CAD build for the part. Positions are in the model's coordinates, mm. Face numbers are marked on the shaded views. A direction names the side the tool comes from. Round coordinates to 2 decimals unless told otherwise and drop trailing zeros. Order: outer loops, then holes, each group sorted by start corner. A loop starts at its lowest first (then second) coordinate and runs counter-clockwise, first axis right, second up. Notation, with made-up numbers: (88, 88) -> (96, 88) arc R20 ccw to (96, 111) -> close; hole circle Ø7 at (81.25, 40.25). An arc over 180 degrees is marked (long way). Return JSON: item names as keys, results as strings. Group by question number.
Q1. Cut at B-B (z = 175). Write the cut outline in (x, y).
Q2. Cut at D-D (y = 35.5). Write the cut outline in (x, z).
Q3. Which spindle directions (+Z, -Z, +X, -X, +Y, -Y) get a long thin tool onto all of the face, cutting with end or side? Do the marked faces 1 and 2. Say none if no direction does.
Q4. Probe line 1 along Z through (x, y) = (81.5, 26.5); line 2 along Z through (x, y) = (73, 26); line 3 along Z through (x, y) = (8.5, 20.5). List the from-to ranges inside material, lowest first.
Q5. Cut at C-C (x = 56). Write the cut outline in (y, z), then the cut area to 3 significant figures.
Q6. Cut at A-A (z = 201.5). Write the cut outline in (x, y).
Q7. Flat gauge pins, fed straight in: pin 1 (3 mm diameter, centred on y = 29, z = 156.5, fed in from +X); pin 2 (1.5 mm diameter, centred on x = 9, y = 27, fed in from +Z); pin 3 (2 mm diameter, centred on x = 36, z = 187.5, fed in from -Y). Where does each tip first touch, or does it go through?
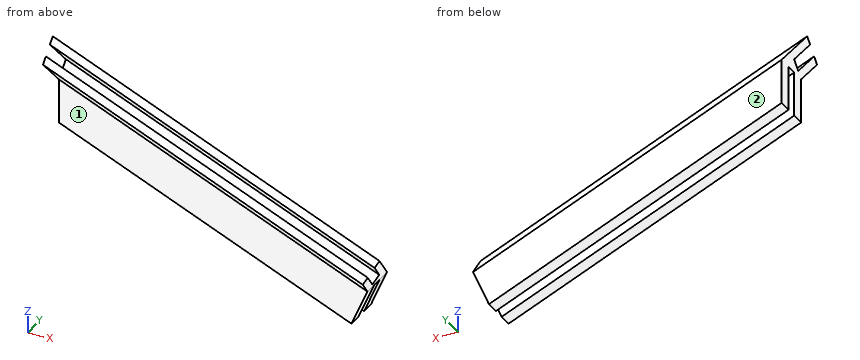
from build123d import *

# Parameters (mm, degrees)
SKETCH1_W           = 214.089522673
SKETCH1_H           = 271.033566845
BOSS_EXTRUDE1_DEPTH = 10
SKETCH3_W           = 107.044761337
SKETCH3_H           = 271.033566845
CUT_EXTRUDE1_DEPTH  = 252.253590179
CUT_EXTRUDE2_DEPTH  = 249.55642867
BOSS_EXTRUDE3_DEPTH = 40
CUT_EXTRUDE3_START  = -165.689856025
CUT_EXTRUDE3_DEPTH  = 205.862728092
CUT_EXTRUDE4_DEPTH  = 250.960593361
CUT_EXTRUDE5_DEPTH  = 250.960593361
CUT_EXTRUDE11_DEPTH = 252.67545035
SKETCH26_W          = 104.148686
SKETCH26_H          = 11.3
BOSS_EXTRUDE7_DEPTH = 45
CUT_EXTRUDE12_DEPTH = 250.816831154
CUT_EXTRUDE13_DEPTH = 252.67545035
CUT_EXTRUDE14_DEPTH = 237.436663672


with BuildPart() as part:
    # Sketch1 → Boss-Extrude1 (new body)
    with BuildSketch(Plane(origin=(0, 0, 0), x_dir=(1, 0, 0), z_dir=(0, 1, 0))):
        with Locations((-3.148375333, -90.062114546)):
            Rectangle(SKETCH1_W, SKETCH1_H)
    extrude(amount=BOSS_EXTRUDE1_DEPTH)

    # Sketch3 → Cut-Extrude1 (cut, through all)
    with BuildSketch(Plane(origin=(0, 10, 0), x_dir=(1, 0, 0), z_dir=(0, 1, 0))):
        with Locations((-56.670756002, -90.062114546)):
            Rectangle(SKETCH3_W, SKETCH3_H)
    extrude(amount=-CUT_EXTRUDE1_DEPTH, mode=Mode.SUBTRACT)

    # Sketch4 → Cut-Extrude2 (cut, through all)
    with BuildSketch(Plane(origin=(0, 10, 0), x_dir=(1, 0, 0), z_dir=(0, 1, 0))):
        Polygon((103.896386003, -181.239506042), (100.834918545, -173.848469781), (9.996584241, 45.454668877), (103.896386003, 45.454668877), align=None)
    extrude(amount=-CUT_EXTRUDE2_DEPTH, mode=Mode.SUBTRACT)

    # Sketch6 → Boss-Extrude3 (add, along a direction that is not the sketch's normal)
    with BuildSketch(Plane(origin=(0, 10, 0), x_dir=(1, 0, 0), z_dir=(0, 1, 0))):
        Polygon((99.572063218, -170.799667324), (103.896386003, -181.239506042), (-3.148375333, -225.578897968), (-3.148375333, -213.347866105), align=None)
    extrude(amount=BOSS_EXTRUDE3_DEPTH, dir=(-0.2705980500730979, 0.7071067811865489, -0.6532814824381872))

    # Cut-Extrude3: read off the stored shape, not the designer's step
    # Cut-Extrude3 outline → Cut-Extrude3 (cut)
    with BuildSketch(Plane(origin=(0, 0, 0), x_dir=(1, 0, 0), z_dir=(0, 0.6785983445458481, -0.7345095552677544)).offset(CUT_EXTRUDE3_START)):
        Polygon((-3.148375333, -165), (-3.148375333, -152.122604304), (-13.972297336, -155.165042499), (-15, -155.45391393), (-15, -165), align=None)
    extrude(amount=CUT_EXTRUDE3_DEPTH, mode=Mode.SUBTRACT)

    # Sketch8 → Cut-Extrude4 (cut, through all)
    with BuildSketch(Plane(origin=(0, 10, 0), x_dir=(1, 0, 0), z_dir=(0, 1, 0))):
        Polygon((-3.148375333, -225.578897968), (103.896386003, -181.239506042), (103.896386003, -225.578897968), align=None)
    extrude(amount=-CUT_EXTRUDE4_DEPTH, mode=Mode.SUBTRACT)

    # Sketch9 → Cut-Extrude5 (cut, through all)
    with BuildSketch(Plane(origin=(0, 10, 0), x_dir=(1, 0, 0), z_dir=(0, 1, 0))):
        Polygon((-3.148375333, -213.347866105), (99.572063218, -170.799667324), (9.996584241, 45.454668877), (-3.148375333, 45.454668877), align=None)
    extrude(amount=-CUT_EXTRUDE5_DEPTH, mode=Mode.SUBTRACT)

    # Sketch25 → Cut-Extrude11 (cut, through all)
    with BuildSketch(Plane(origin=(24.603270673, 0, -10.191008392), x_dir=(-0.38268343236508967, 0, -0.9238795325112868), z_dir=(0.9238795325112867, 0, -0.3826834323650896))):
        Polygon((-178.918624473, 38.284271247), (-178.918624473, 26.984271247), (-167.618624473, 38.284271247), align=None)
    extrude(amount=-CUT_EXTRUDE11_DEPTH, mode=Mode.SUBTRACT)

    # Sketch26 → Boss-Extrude7 (add)
    with BuildSketch(Plane(origin=(68.469193327, 0, 165.299255136), x_dir=(-0.9238795325112868, 0, 0.3826834323650896), z_dir=(-0.38268343236508956, 0, -0.9238795325112867))):
        with Locations((25.443954722, 32.634271247)):
            Rectangle(SKETCH26_W, SKETCH26_H)
    extrude(amount=BOSS_EXTRUDE7_DEPTH)

    # Sketch27 → Cut-Extrude12 (cut, through all)
    with BuildSketch(Plane.XZ.offset(-26.984271247)):
        Polygon((-3.148375333, 194.964223379), (-3.148375333, 146.256574366), (-20.36912979, 153.389644416), align=None)
    extrude(amount=-CUT_EXTRUDE12_DEPTH, mode=Mode.SUBTRACT)

    # Sketch29 → Cut-Extrude13 (cut, through all)
    with BuildSketch(Plane(origin=(24.603270673, 0, -10.191008392), x_dir=(-0.38268343236508967, 0, -0.9238795325112868), z_dir=(0.9238795325112867, 0, -0.3826834323650896))):
        Polygon((-188.111012628, 17.791883092), (-189.772713564, 19.453584028), (-180.580325409, 28.645972183), (-182.906923537, 30.972570312), (-192.099311693, 21.780182156), (-193.761012628, 23.441883092), (-207.20289572, 10), (-207.20289572, 0), (-195.90289572, 0), (-195.90289572, 10), align=None)
    extrude(amount=-CUT_EXTRUDE13_DEPTH, mode=Mode.SUBTRACT)

    # Sketch31 → Cut-Extrude14 (cut, through all)
    with BuildSketch(Plane(origin=(24.603270673, 0, -10.191008392), x_dir=(-0.38268343236508967, 0, -0.9238795325112868), z_dir=(0.9238795325112867, 0, -0.3826834323650896))):
        Polygon((-133.918624473, 38.284271247), (-165.918624473, 38.284271247), (-165.918624473, 34.284271247), (-178.918624473, 34.284271247), (-178.918624473, 30.984271247), (-165.918624473, 30.984271247), (-165.918624473, 26.984271247), (-133.918624473, 26.984271247), align=None)
    extrude(amount=-CUT_EXTRUDE14_DEPTH, mode=Mode.SUBTRACT)


solid = part.part
Solution:
{
 "1": {"outline": "(11.08, 26.98) -> (45.05, 26.98) -> (69.07, 17.79) -> (73.41, 19.45) -> (49.39, 28.65) -> (55.47, 30.97) -> (79.49, 21.78) -> (83.83, 23.44) -> (45.05, 38.28) -> (11.08, 38.28) -> (11.08, 34.28) -> (45.05, 34.28) -> (45.05, 30.98) -> (11.08, 30.98) -> close"},
 "2": {"outline": "(-3.15, 180.89) -> (88.1, 143.1) -> (94.14, 157.68) -> (-3.15, 197.98) -> close"},
 "3": {"face 1": "-Z, -X, -Y", "face 2": "+Z, -Z, +X, -X, +Y"},
 "4": {"line 1": "z = 160.43 to 164.02, 169.06 to 172.66", "line 2": "z = 164.49 to 168.09, 173.12 to 176.72", "line 3": "z = 197.16 to 200.76"},
 "5": {"outline": "(17.79, 180.41) -> (26.98, 170.46) -> (26.98, 156.39) -> (30.98, 156.39) -> (30.98, 170.46) -> (34.28, 170.46) -> (34.28, 156.39) -> (38.28, 156.39) -> (38.28, 170.46) -> (23.44, 186.53) -> (21.78, 184.73) -> (30.97, 174.78) -> (28.65, 172.26) -> (19.45, 182.21) -> close", "area": "213 mm²"},
 "6": {"outline": "(-3.15, 20.95) -> (5.09, 17.79) -> (9.44, 19.45) -> (-3.15, 24.27) -> close; (-3.15, 28.92) -> (15.52, 21.78) -> (19.86, 23.44) -> (-3.15, 32.25) -> close"},
 "7": {"pin 1": "stops at x = 94.16", "pin 2": "stops at z = 203.02", "pin 3": "stops at y = 17.9"}
}
